Could you check a few things on this drawing? It's one solid part, dimensions in mm from its lowest x, y, z. A direction names the side the tool comes from. Round coordinates to 2 decimals unless told otherwise and drop trailing zeros. Loops run counter-clockwise (first coordinate to the right, second up) from the corner with the lowest first, then second, coordinate; pieces in that order, holes last. Notation, with made-up numbers: (-10, 44.25) -> (41, 44.25) arc R17 cw to (41, 53.25) -> close; hole circle Ø7 at (72, 28.25). An arc over 180 degrees is marked (long way). Put each result on its own line as item: value. Start each with the question number.
1. Imagine slicing it at A-A, the plane z = 7.5. Please give me the cut outline in (x, y).
2. I need wall thicknesses on line 1 (X direction, y = 19, z = 8.25); line 2 (Z direction, x = 2.3, y = 13); line 3 (Z direction, x = 9, y = 14). Which ranges of each line are inside material? Lowest first, please. Write a range as [from, to].
3. I'm going to push flat-ended pins straight in: P1, Ø5, axis at x = 6, z = 11, coming from the +Y side; P2, Ø2, axis at x = 5, z = 13.5, coming from the -Y side; P3, Ø7, axis at y = 13, z = 7.5, coming from the -X side; P4, Ø1.8, axis at x = 7.5, z = 9.5, coming from the +Y side. Where does each tip first touch, or does it pass through?
4. Imagine slicing it at C-C, the plane y = 11.75. Please give me the cut outline in (x, z), and give its area (3 significant figures).
5. Imagine slicing it at D-D, the plane z = 12. Please give me the cut outline in (x, y), and give its area (3 significant figures).
6. If we mould it in two halves opening along X, with no side actions, what happens to the marked faces 1, 2 and 3? For each: pulls with the +X half, pulls with the -X half, needs draft (parallel to the pull), parting line crosses it, or undercut.
7. Imagine slicing it at B-B, the plane x = 12. Please give me the cut outline in (y, z).
8. Which directions (+Z, -Z, +X, -X, +Y, -Y) give clear straight access to the entire face, cutting with the end or side of a thin tool? Please do the marked faces 4 and 5.
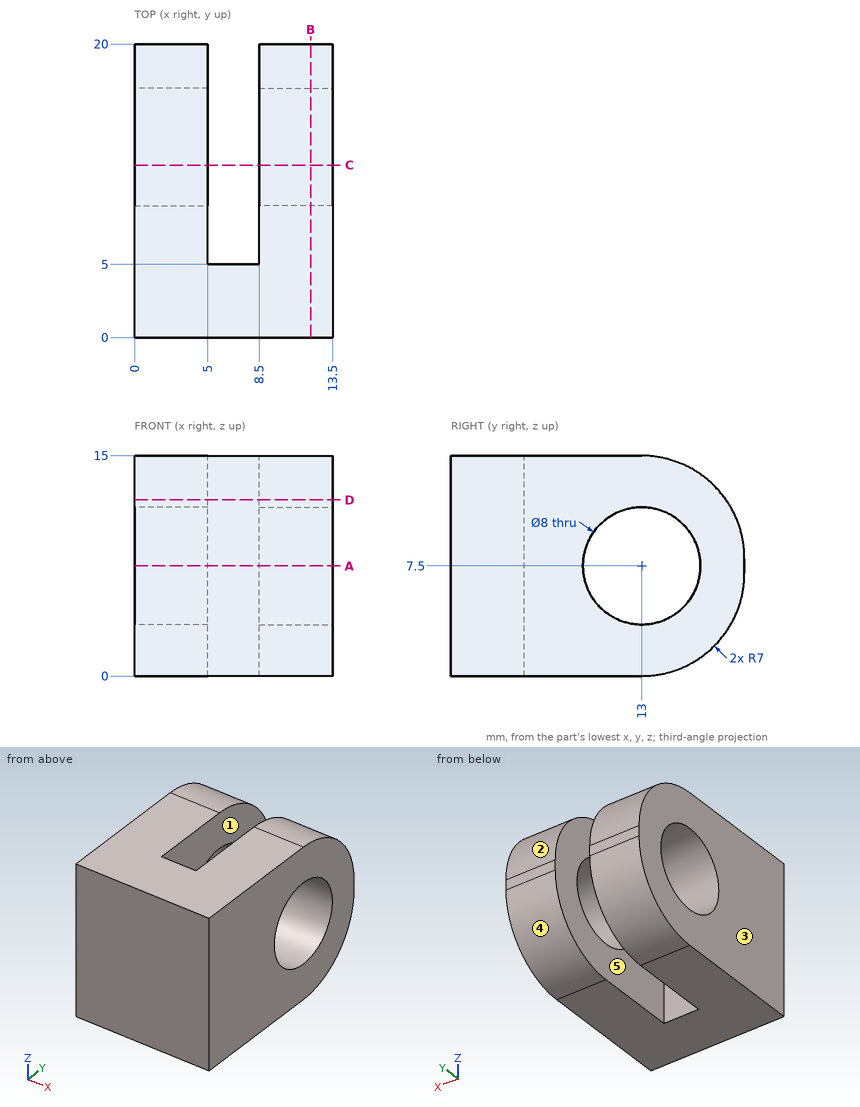
Entries:
1. outline: (0, 0) -> (13.5, 0) -> (13.5, 9) -> (8.5, 9) -> (8.5, 5) -> (5, 5) -> (5, 9) -> (0, 9) -> close; (0, 17) -> (5, 17) -> (5, 20) -> (0, 20) -> close; (8.5, 17) -> (13.5, 17) -> (13.5, 20) -> (8.5, 20) -> close
2. line 1: [0, 5], [8.5, 13.5]
2. line 2: [0, 3.5], [11.5, 15]
2. line 3: [0.07, 3.63], [11.37, 14.93]
3. P1: y = 19.96
3. P2: y = 0
3. P3: through
3. P4: y = 5
4. outline: (0, 0) -> (5, 0) -> (5, 3.7) -> (0, 3.7) -> close; (0, 11.3) -> (5, 11.3) -> (5, 15) -> (0, 15) -> close; (8.5, 0) -> (13.5, 0) -> (13.5, 3.7) -> (8.5, 3.7) -> close; (8.5, 11.3) -> (13.5, 11.3) -> (13.5, 15) -> (8.5, 15) -> close
4. area: 74.0 mm^2
5. outline: (0, 0) -> (13.5, 0) -> (13.5, 18.74) -> (8.5, 18.74) -> (8.5, 5) -> (5, 5) -> (5, 18.74) -> (0, 18.74) -> close
5. area: 205 mm^2
6. face 1: undercut
6. face 2: needs draft
6. face 3: pulls with the -X half
7. outline: (0, 0) -> (13, 0) arc R7 ccw to (20, 7) -> (20, 8) arc R7 ccw to (13, 15) -> (0, 15) -> close; hole circle Ø8 at (13, 7.5)
8. face 4: -Z, +X, -X, +Y
8. face 5: +Z, -Z, +Y
